from build123d import *

# Parameters (mm, degrees)
SKETCH_1_W               = 30
SKETCH_1_H               = 25
EXTRUDE_1_DEPTH          = 30
CUT_EXTRUDE_START        = -25
CUT_EXTRUDE_1_DEPTH      = 25
CUT_EXTRUDE_START_2      = -30
CUT_EXTRUDE_2_DEPTH      = 30
CUT_EXTRUDE_3_DEPTH      = 45.229515196
CUT_EXTRUDE_3_DEPTH_BACK = 45.229515196
CUT_EXTRUDE_4_DEPTH      = 45.229515196
CUT_EXTRUDE_4_DEPTH_BACK = 45.229515196
SHELL_2_T                = -1.8
SKETCH_8_W               = 40
SKETCH_8_H               = 20
SKETCH_8_W_2             = 26.4
SKETCH_8_H_2             = 16.4
EXTRUDE_2_DEPTH          = 2
EXTRUDE_3_DEPTH          = 15
EXTRUDE_3_DEPTH_BACK     = 2
SKETCH_9_W               = 40
SKETCH_9_H               = 2
SKETCH_10_W              = 2
SKETCH_10_H              = 17
EXTRUDE_4_DEPTH          = 8
CUT_EXTRUDE_5_REACH      = 66.15
SKETCH_13_R              = 1.7
CUT_EXTRUDE_6_REACH      = 59.602
SKETCH_14_R              = 1.7


# Read off the part's stored shape, not the designer's step: 切除-拉伸1, 切除-拉伸2
with BuildPart() as part:
    # 草图1 → 凸台-拉伸1 (new body)
    with BuildSketch(Plane(origin=(0, 0, 0), x_dir=(1, 0, 0), z_dir=(0, 1, 0))):
        Rectangle(SKETCH_1_W, SKETCH_1_H)
    extrude(amount=EXTRUDE_1_DEPTH)

    # 切除-拉伸1 outline → 切除-拉伸1 (cut)
    with BuildSketch(Plane(origin=(0, 0, -12.5), x_dir=(-1, 0, 0), z_dir=(0, 0, -1)).offset(CUT_EXTRUDE_START)):
        with BuildLine():
            add(Edge.make_bspline(
                [(-15, 25), (-6.511377405, 22.051776189), (-3.763777339, 18.136586702), (-1, 0)],
                knots=[0, 0, 0, 0, 1, 1, 1, 1], degree=3))
            Line((-15, 25), (-15, 0))
            Line((-15, 0), (-1, 0))
        make_face()
    extrude(amount=CUT_EXTRUDE_1_DEPTH, mode=Mode.SUBTRACT)

    # 切除-拉伸2 outline → 切除-拉伸2 (cut)
    with BuildSketch(Plane.ZY.offset(15).offset(CUT_EXTRUDE_START_2)):
        with BuildLine():
            add(Edge.make_bspline(
                [(-7.5, 30), (-7.5, 23.858714032), (-8.903080152, 17.199411136), (-12.5, 10)],
                knots=[0, 0, 0, 0, 1, 1, 1, 1], degree=3))
            Line((-7.5, 30), (-12.5, 30))
            Line((-12.5, 30), (-12.5, 10))
        make_face()
    extrude(amount=CUT_EXTRUDE_2_DEPTH, mode=Mode.SUBTRACT)

    # 草图6 → 切除-拉伸3 (cut, two sides: drawn at the far end of the back side and taken through both)
    with BuildSketch(Plane.ZY.offset(15).offset(-CUT_EXTRUDE_3_DEPTH_BACK)):
        with BuildLine():
            Line((34.396469071, 110.338119425), (12.5, 25))
            ThreePointArc((12.5, 25), (3.420693976, 9.079306024), (-12.5, 0))
            Line((-12.5, 0), (-97.838119425, -21.896469071))
            Line((-97.838119425, -21.896469071), (26.757626769, -146.492215265))
            Line((26.757626769, -146.492215265), (158.992215265, -14.257626769))
            Line((158.992215265, -14.257626769), (34.396469071, 110.338119425))
        make_face()
    extrude(amount=CUT_EXTRUDE_3_DEPTH + CUT_EXTRUDE_3_DEPTH_BACK, mode=Mode.SUBTRACT)

    # 草图7 → 切除-拉伸4 (cut, two sides: drawn at the far end of the back side and taken through both)
    with BuildSketch(Plane.ZY.offset(15).offset(-CUT_EXTRUDE_4_DEPTH_BACK)):
        Polygon((-34.201614467, 90.991527796), (-12.5, 10), (-10.017865444, 0.736547724), (11.683749023, -80.254980072), (-150.299306569, -123.658209006), (-196.184670059, 47.588298863), align=None)
    extrude(amount=CUT_EXTRUDE_4_DEPTH + CUT_EXTRUDE_4_DEPTH_BACK, mode=Mode.SUBTRACT)

    # 抽壳2
    shell_2_openings = [part.faces().sort_by_distance(p)[0] for p in [
        (0, 30, 2.5),
        (-6.528277813, 5.44772403, -11.28022133),
    ]]
    offset(amount=SHELL_2_T, openings=shell_2_openings)

    # 草图8 → 凸台-拉伸2 (add)
    with BuildSketch(Plane(origin=(0, 30, 0), x_dir=(1, 0, 0), z_dir=(0, 1, 0))):
        with Locations((5, -2.5)):
            Rectangle(SKETCH_8_W, SKETCH_8_H)
        with Locations((0, -2.5)):
            Rectangle(SKETCH_8_W_2, SKETCH_8_H_2, mode=Mode.SUBTRACT)
    extrude(amount=EXTRUDE_2_DEPTH)

    # 草图9 → 凸台-拉伸3 (add, two sides: drawn at the far end of the back side and taken through both)
    with BuildSketch(Plane(origin=(0, 32, 0), x_dir=(1, 0, 0), z_dir=(0, 1, 0)).offset(-EXTRUDE_3_DEPTH_BACK)):
        with Locations((5, 8.5)):
            Rectangle(SKETCH_9_W, SKETCH_9_H)
    extrude(amount=EXTRUDE_3_DEPTH + EXTRUDE_3_DEPTH_BACK)

    # 草图10 → 凸台-拉伸4 (add)
    with BuildSketch(Plane(origin=(0, 0, -9.5), x_dir=(-1, 0, 0), z_dir=(0, 0, -1))):
        with Locations((14, 38.5)):
            Rectangle(SKETCH_10_W, SKETCH_10_H)
    extrude(amount=EXTRUDE_4_DEPTH)

    # 草图13 → 切除-拉伸5 (cut, up to next)
    with BuildSketch(Plane.ZY.offset(15), mode=Mode.PRIVATE) as cut_extrude_5_sk1:
        with Locations((-13.5, 43)):
            Circle(SKETCH_13_R)
    cut_extrude_5_tool1 = extrude(cut_extrude_5_sk1.sketch, amount=-CUT_EXTRUDE_5_REACH, mode=Mode.PRIVATE) & part.part
    # 草图13 → 切除-拉伸5 (cut, up to next)
    with BuildSketch(Plane.ZY.offset(15), mode=Mode.PRIVATE) as cut_extrude_5_sk2:
        with Locations((-13.5, 35)):
            Circle(SKETCH_13_R)
    cut_extrude_5_tool2 = extrude(cut_extrude_5_sk2.sketch, amount=-CUT_EXTRUDE_5_REACH, mode=Mode.PRIVATE) & part.part
    add(cut_extrude_5_tool1.solids().sort_by_distance((-15, 43, -13.5))[0], mode=Mode.SUBTRACT)
    add(cut_extrude_5_tool2.solids().sort_by_distance((-15, 35, -13.5))[0], mode=Mode.SUBTRACT)

    # 草图14 → 切除-拉伸6 (cut, up to next)
    with BuildSketch(Plane(origin=(0, 0, -9.5), x_dir=(-1, 0, 0), z_dir=(0, 0, -1)), mode=Mode.PRIVATE) as cut_extrude_6_sk1:
        with Locations((-22, 35)):
            Circle(SKETCH_14_R)
    cut_extrude_6_tool1 = extrude(cut_extrude_6_sk1.sketch, amount=-CUT_EXTRUDE_6_REACH, mode=Mode.PRIVATE) & part.part
    add(cut_extrude_6_tool1.solids().sort_by_distance((22, 35, -9.5))[0], mode=Mode.SUBTRACT)


solid = part.part
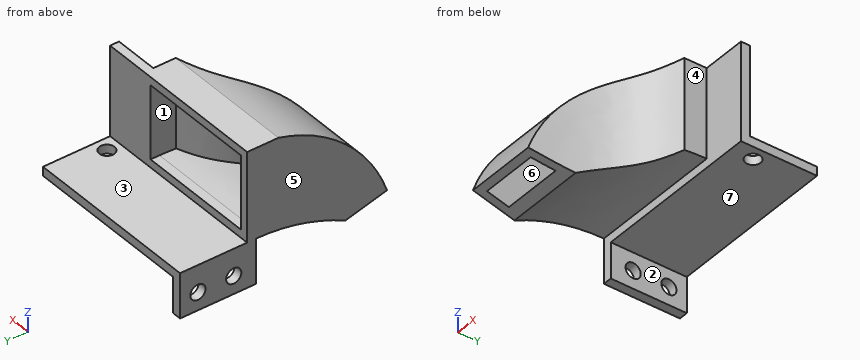
Geometry check sheet. Reference: the model listing, model coordinates, mm. Face numbers are marked on the shaded views. A direction names the side the tool comes from. Give positions to 0.01 mm unless a question says otherwise; leave off trailing zeros. Loops run counter-clockwise (first coordinate to the right, second up) from the corner with the lowest first, then second, coordinate; pieces in that order, holes last.
(1) Depth check by flat-ended pin: pin 1 Ø8 at (x, z) = (-2, -0.5) entering from -Y; pin 2 Ø4.5 at (x, y) = (12, 37) entering from +Z; pin 3 Ø1.5 at (x, z) = (21, -8) entering from -Y; pin 4 Ø8 at (x, z) = (2.5, -10) entering from -Y. Enter the tip coordinate at first touch or a pass-through.
From the geometry:
pin 1: stops at y = 3.15
pin 2: stops at z = -7.5
pin 3: stops at y = 30
pin 4: stops at y = 0.74
(2) Thickness scan on L1, parallel to Y at x = -13.9, z = -13.5; L2, parallel to Y at x = 16, z = 8; L3, parallel to X at y = 23, z = -4. Record the ranges inside material, lowest first.
From the geometry:
L1: y = 30 to 33.3, 36.7 to 41.3, 44.7 to 47
L2: y = 30 to 32
L3: x = -15 to -13.2, 7.47 to 10.53
(3) Set-up check for the marked faces 1, 2, 3 and 4: record each of +Z, -Z, +X, -X, +Y, -Y from which the full face is reachable in a straight line by a thin tool's end or side.
From the geometry:
face 1: +Y
face 2: -Z, +X, +Y
face 3: +Z, +X, -X, +Y
face 4: +Z, -Z, +X, -Y
(4) Section check C-C on y = 43. Record the cut outline in (x, z).
From the geometry:
outline: (-15, -17.5) - (-13, -17.5) - (-13, -15.2) - (-15, -15.2) - close; (-15, -11.8) - (-13, -11.8) - (-13, -9.5) - (25, -9.5) - (25, -7.5) - (-15, -7.5) - close
(5) Section check A-A on z = -13.5. Record the cut outline in (x, y), then the cut area to 3 significant figures.
From the geometry:
outline: (-15, 30) - (-13, 30) - (-13, 33.3) - (-15, 33.3) - close; (-15, 36.7) - (-13, 36.7) - (-13, 41.3) - (-15, 41.3) - close; (-15, 44.7) - (-13, 44.7) - (-13, 47) - (-15, 47) - close
area: 20.4 mm2
(6) Section check B-B on x = 22. Record the cut outline in (y, z), then the cut area to 3 significant figures.
From the geometry:
outline: (30, -9.5) - (33.3, -9.5) - (33.3, -7.5) - (32, -7.5) - (32, 12.5) - (30, 12.5) - close; (36.7, -9.5) - (47, -9.5) - (47, -7.5) - (36.7, -7.5) - close
area: 67.2 mm2
(7) Section check D-D on y = 36. Record the cut outline in (x, z).
From the geometry:
outline: (-15, -17.5) - (-13, -17.5) - (-13, -14.87) - (-15, -14.87) - close; (-15, -12.13) - (-13, -12.13) - (-13, -9.5) - (20.63, -9.5) - (20.63, -7.5) - (-15, -7.5) - close; (23.37, -9.5) - (25, -9.5) - (25, -7.5) - (23.37, -7.5) - close
(8) Release check for a two-part mould opening along X. For the marked faces 5, 6 and 7 record: released by +X, released by -X, zero draft, split by the parting line, or undercut.
From the geometry:
face 5: released by -X
face 6: undercut
face 7: zero draft
